from build123d import *

# Parameters (mm, degrees)
SKETCH_2_R      = 1.5
EXTRUDE_1_DEPTH = 1.5
SKETCH_3_R      = 17.5
EXTRUDE_2_DEPTH = 33
SKETCH_4_W      = 21
SKETCH_4_H      = 20
EXTRUDE_3_DEPTH = 15
FILLET_1_R      = 10


with BuildPart() as part:
    # 草图2 → 凸台-拉伸1 (new body)
    with BuildSketch(Plane(origin=(0, 0, 0), x_dir=(1, 0, 0), z_dir=(0, 1, 0))):
        with BuildLine():
            Line((255.573084798, 167.040097328), (242.323084798, 167.040097328))
            Line((242.323084798, 167.040097328), (234.323084798, 159.040097328))
            Line((234.323084798, 159.040097328), (234.323084798, 157.622673023))
            ThreePointArc((234.323084798, 157.622673023), (236.506384931, 155.778710115), (237.323084798, 153.040097328))
            ThreePointArc((237.323084798, 153.040097328), (236.506384931, 150.30148454), (234.323084798, 148.457521633))
            Line((234.323084798, 148.457521633), (234.323084798, 144.040097328))
            Line((234.323084798, 144.040097328), (237.323084798, 144.040097328))
            Line((237.323084798, 144.040097328), (237.323084798, 108.040097328))
            Line((237.323084798, 108.040097328), (234.323084798, 108.040097328))
            Line((234.323084798, 108.040097328), (234.323084798, 104.622673023))
            ThreePointArc((234.323084798, 104.622673023), (236.506384931, 102.778710115), (237.323084798, 100.040097328))
            ThreePointArc((237.323084798, 100.040097328), (236.506384931, 97.30148454), (234.323084798, 95.457521633))
            Line((234.323084798, 95.457521633), (234.323084798, 89.040097328))
            Line((234.323084798, 89.040097328), (254.323084798, 63.040097328))
            Line((254.323084798, 63.040097328), (273.323084798, 63.040097328))
            Line((273.323084798, 63.040097328), (271.323084798, 81.040097328))
            Line((271.323084798, 81.040097328), (291.434195909, 83.040097328))
            Line((291.434195909, 83.040097328), (294.323084798, 57.040097328))
            Line((294.323084798, 57.040097328), (324.323084798, 57.040097328))
            Line((324.323084798, 57.040097328), (327.211973687, 83.040097328))
            Line((327.211973687, 83.040097328), (347.323084798, 81.040097328))
            Line((347.323084798, 81.040097328), (345.323084798, 63.040097328))
            Line((345.323084798, 63.040097328), (364.323084798, 63.040097328))
            Line((364.323084798, 63.040097328), (384.323084798, 89.040097328))
            Line((384.323084798, 89.040097328), (384.323084798, 95.457521633))
            ThreePointArc((384.323084798, 95.457521633), (381.323084798, 100.040097328), (384.323084798, 104.622673023))
            Line((384.323084798, 104.622673023), (384.323084798, 108.040097328))
            Line((384.323084798, 108.040097328), (381.323084798, 108.040097328))
            Line((381.323084798, 108.040097328), (381.323084798, 144.040097328))
            Line((381.323084798, 144.040097328), (384.323084798, 144.040097328))
            Line((384.323084798, 144.040097328), (384.323084798, 148.457521633))
            ThreePointArc((384.323084798, 148.457521633), (381.323084798, 153.040097328), (384.323084798, 157.622673023))
            Line((384.323084798, 157.622673023), (384.323084798, 159.040097328))
            Line((384.323084798, 159.040097328), (376.323084798, 167.040097328))
            Line((376.323084798, 167.040097328), (363.073084798, 167.040097328))
            Line((363.073084798, 167.040097328), (363.073084798, 164.040097328))
            Line((363.073084798, 164.040097328), (327.073084798, 164.040097328))
            Line((327.073084798, 164.040097328), (327.073084798, 167.040097328))
            Line((327.073084798, 167.040097328), (320.573084798, 167.040097328))
            Line((320.573084798, 167.040097328), (320.573084798, 164.040097328))
            Line((320.573084798, 164.040097328), (298.073084798, 164.040097328))
            Line((298.073084798, 164.040097328), (298.073084798, 167.040097328))
            Line((298.073084798, 167.040097328), (291.573084798, 167.040097328))
            Line((291.573084798, 167.040097328), (291.573084798, 164.040097328))
            Line((291.573084798, 164.040097328), (255.573084798, 164.040097328))
            Line((255.573084798, 164.040097328), (255.573084798, 167.040097328))
        make_face()
        with Locations(Location((239.323084798, 105.052003777, 0), (0, 0, 270))):
            Circle(SKETCH_2_R, mode=Mode.SUBTRACT)
        with Locations(Location((379.323084798, 105.052003777, 0), (0, 0, 270))):
            Circle(SKETCH_2_R, mode=Mode.SUBTRACT)
        with Locations(Location((238.323084798, 147.040097328, 0), (0, 0, 270))):
            Circle(SKETCH_2_R, mode=Mode.SUBTRACT)
        with Locations(Location((380.323084798, 147.040097328, 0), (0, 0, 270))):
            Circle(SKETCH_2_R, mode=Mode.SUBTRACT)
    extrude(amount=EXTRUDE_1_DEPTH)

    # 草图3 → 凸台-拉伸2 (add)
    with BuildSketch(Plane(origin=(0, 1.5, 0), x_dir=(1, 0, 0), z_dir=(0, 1, 0))):
        with Locations(Location((275.323084798, 141.040097328, 0), (0, 0, 270))):
            Circle(SKETCH_3_R)
        with Locations(Location((343.323084798, 141.040097328, 0), (0, 0, 270))):
            Circle(SKETCH_3_R)
        with Locations(Location((275.323084798, 105.040097328, 0), (0, 0, 270))):
            Circle(SKETCH_3_R)
        with Locations(Location((343.323084798, 105.040097328, 0), (0, 0, 270))):
            Circle(SKETCH_3_R)
    extrude(amount=EXTRUDE_2_DEPTH)

    # 草图4 → 凸台-拉伸3 (add)
    with BuildSketch(Plane.XZ):
        with Locations((357.823084798, -77.040097328)):
            Rectangle(SKETCH_4_W, SKETCH_4_H)
    extrude(amount=EXTRUDE_3_DEPTH)

    # 圆角1
    # the kernel refuses this fillet: 10 mm, written as the material it takes off along each edge
    with BuildSketch(Plane(origin=(234.323084798, -8.403282896, -159.040097328), x_dir=(0, 0, 1), z_dir=(0, 1, 0))) as fillet_1_piece_1:
        with BuildLine():
            CenterArc((4.694260484, 9.44787514), FILLET_1_R, 225, 25.871759313)
            Line((-2.376807328, 2.376807328), (-2.518228684, 2.235385972))
            Line((-2.518228684, 2.235385972), (-0.141421356, -0.141421356))
            Line((-0.141421356, -0.141421356), (0, -0.2))
            ThreePointArc((0, -0.2), (0.708712153, -0.2), (1.351887581, -0.188957503))
            Line((1.351887581, -0.188957503), (1.417424305, 0))
        make_face()
    extrude(amount=18.306565791, mode=Mode.SUBTRACT)
    with BuildSketch(Plane(origin=(242.323084798, -10.355339059, -167.040097328), x_dir=(-0.7071067811865476, 0, 0.7071067811865476), z_dir=(0, 1, 0)), Plane(origin=(376.323084798, -10.355339059, -167.040097328), x_dir=(-1, 0, 0), z_dir=(0, 1, 0))) as fillet_1_piece_2:
        with BuildLine():
            CenterArc((FILLET_1_R * 0.414213562373, FILLET_1_R), FILLET_1_R, 225, 45)
            Line((-FILLET_1_R * 0.292893218813, FILLET_1_R * 0.292893218813), (-FILLET_1_R * 0.307035354437, FILLET_1_R * 0.27875108319))
            Line((-FILLET_1_R * 0.307035354437, FILLET_1_R * 0.27875108319), (-FILLET_1_R * 0.00828427124746, -FILLET_1_R * 0.02))
            Line((-FILLET_1_R * 0.00828427124746, -FILLET_1_R * 0.02), (FILLET_1_R * 0.414213562373, -FILLET_1_R * 0.02))
            Line((FILLET_1_R * 0.414213562373, -FILLET_1_R * 0.02), (FILLET_1_R * 0.414213562373, 0))
        make_face()
    extrude(amount=22.210678119, mode=Mode.SUBTRACT)
    with BuildSketch(Plane(origin=(384.323084798, -8.403282896, -159.040097328), x_dir=(-0.7071067811865475, 0, -0.7071067811865475), z_dir=(0, 1, 0))) as fillet_1_piece_3:
        with BuildLine():
            CenterArc((3.361313158, 10), FILLET_1_R, 244.128240687, 25.871759313)
            Line((-1.002270338, 1.002270338), (-1.089542008, 0.822315745))
            ThreePointArc((-1.089542008, 0.822315745), (-0.642556525, 0.359713813), (-0.141421356, -0.141421356))
            Line((-0.141421356, -0.141421356), (0, -0.2))
            Line((0, -0.2), (3.361313158, -0.2))
            Line((3.361313158, -0.2), (3.361313158, 0))
        make_face()
    extrude(amount=18.306565791, mode=Mode.SUBTRACT)
    with BuildSketch(Plane(origin=(384.323084798, -8.503048667, -89.040097328), x_dir=(0, 0, -1), z_dir=(0, 1, 0)), Plane(origin=(234.323084798, -8.503048667, -89.040097328), x_dir=(0.6097107608496891, 0, 0.7926239891046025), z_dir=(0, 1, 0))) as fillet_1_piece_4:
        with BuildLine():
            CenterArc((FILLET_1_R * 0.340121946686, FILLET_1_R), FILLET_1_R, 232.431407971, 37.568592029)
            Line((-FILLET_1_R * 0.269588814164, FILLET_1_R * 0.207376010895), (-FILLET_1_R * 0.281783029381, FILLET_1_R * 0.191523531113))
            Line((-FILLET_1_R * 0.281783029381, FILLET_1_R * 0.191523531113), (-FILLET_1_R * 0.00680243893371, -FILLET_1_R * 0.02))
            Line((-FILLET_1_R * 0.00680243893371, -FILLET_1_R * 0.02), (FILLET_1_R * 0.340121946686, -FILLET_1_R * 0.02))
            Line((FILLET_1_R * 0.340121946686, -FILLET_1_R * 0.02), (FILLET_1_R * 0.340121946686, 0))
        make_face()
    extrude(amount=18.506097334, mode=Mode.SUBTRACT)
    with BuildSketch(Plane(origin=(364.323084798, -12.310037436, -63.040097328), x_dir=(0.6097107608496888, 0, -0.792623989104603), z_dir=(0, 1, 0)), Plane(origin=(254.323084798, -12.310037436, -63.040097328), x_dir=(1, 0, 0), z_dir=(0, 1, 0))) as fillet_1_piece_5:
        with BuildLine():
            CenterArc((FILLET_1_R * 0.492401497451, FILLET_1_R), FILLET_1_R, 217.568592029, 52.431407971)
            Line((-FILLET_1_R * 0.300222491654, FILLET_1_R * 0.39028923915), (-FILLET_1_R * 0.316074971436, FILLET_1_R * 0.378095023933))
            Line((-FILLET_1_R * 0.316074971436, FILLET_1_R * 0.378095023933), (-FILLET_1_R * 0.00984802994901, -FILLET_1_R * 0.02))
            Line((-FILLET_1_R * 0.00984802994901, -FILLET_1_R * 0.02), (FILLET_1_R * 0.492401497451, -FILLET_1_R * 0.02))
            Line((FILLET_1_R * 0.492401497451, -FILLET_1_R * 0.02), (FILLET_1_R * 0.492401497451, 0))
        make_face()
    extrude(amount=26.120074873, mode=Mode.SUBTRACT)
    with BuildSketch(Plane(origin=(324.323084798, -22.376069828, -57.040097328), x_dir=(0.1104315260748475, 0, -0.9938837346736189), z_dir=(0, 1, 0)), Plane(origin=(294.323084798, -22.376069828, -57.040097328), x_dir=(1, 0, 0), z_dir=(0, 1, 0))) as fillet_1_piece_6:
        with BuildLine():
            CenterArc((FILLET_1_R * 0.895042793126, FILLET_1_R), FILLET_1_R, 186.340191746, 83.659808254)
            Line((-FILLET_1_R * 0.0988409415472, FILLET_1_R * 0.889568473925), (-FILLET_1_R * 0.118718616241, FILLET_1_R * 0.887359843404))
            Line((-FILLET_1_R * 0.118718616241, FILLET_1_R * 0.887359843404), (-FILLET_1_R * 0.0179008558625, -FILLET_1_R * 0.02))
            Line((-FILLET_1_R * 0.0179008558625, -FILLET_1_R * 0.02), (FILLET_1_R * 0.895042793126, -FILLET_1_R * 0.02))
            Line((FILLET_1_R * 0.895042793126, -FILLET_1_R * 0.02), (FILLET_1_R * 0.895042793126, 0))
        make_face()
    extrude(amount=46.252139656, mode=Mode.SUBTRACT)


solid = part.part
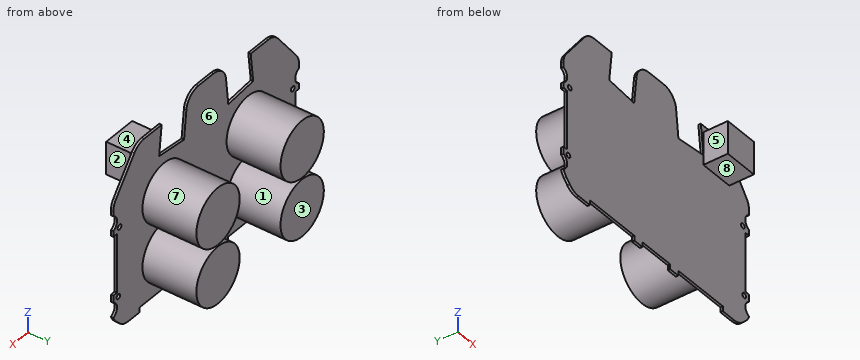
The listing builds one solid part. Answer for the finished solid, in the listing's coordinates (mm). Face numbers are marked on the shaded views. A direction names the side the tool comes from. Coordinates: 2 decimals unless noted, no trailing zeros. Loops run counter-clockwise (first coordinate to the right, second up) from the corner with the lowest first, then second, coordinate; pieces in that order, holes last. Notation, with made-up numbers: (-6.75, -11) -> (14.25, -11) arc R30 ccw to (14.25, 24) -> close; hole circle Ø11 at (50, 30). An arc over 180 degrees is marked (long way). Write item = value, one per line. Start each with the question number.
1) Straight lines are drawn through the part: line 1 (Y direction, x = 262, z = -161.5); line 2 (X direction, y = 2.5, z = -157); line 3 (X direction, y = 5, z = -140). For each, find the intervals that lie inside material, in ascending order. Write a range as from..to.
2) A cutting plane is placed at C-C (y = 8). Give the vertices of the cut face in (x, z), then the cut area to 3 significant figures.
3) A cutting plane is placed at A-A (x = 357.5). Give the vertices of the cut face in (y, z).
4) Given pin 1 Ø0.8 at (x, y) = (235.5, 1) entering from +Z; pin 2 Ø4 at (x, z) = (239.32, -105.05) entering from +Y; pin 3 Ø1.6 at (y, z) = (1, -119) entering from -X, each flat-ended and moving along its own axis, determine where each tip first touches the part or whether it passes through.
5) A cutting plane is placed at D-D (y = -4). Give the vertices of the cut face in (x, z).
6) A tool of negligible diameter and unlimited length cuts with its end or side. For the marked faces 1, 2, 3 and 4, from which of +Z, -Z, +X, -X, +Y, -Y can it reach the whole face along a straight path? Write none if from no direction.
7) A cutting plane is placed at B-B (z = -129). Give the vertices of the cut face in (x, y).
8) The mould has two halves that part along X. Classify the marked faces 5, 6, 7 and 8: released by +X, released by -X, zero draft, split by the parting line, or undercut.
Responses:
q1.line_1 = 0..1.5
q1.line_2 = 268.14..282.5, 336.14..350.5
q1.line_3 = 257.85..292.79, 325.85..360.79
q2.outline = circle Ø35 at (275.32, -141.04); circle Ø35 at (275.32, -105.04); circle Ø35 at (343.32, -141.04); circle Ø35 at (343.32, -105.04)
q2.area = 3,850 mm²
q3.outline = (-15, -87.04) -> (0, -87.04) -> (0, -164.04) -> (1.5, -164.04) -> (1.5, -151.3) -> (34.5, -151.3) -> (34.5, -130.78) -> (1.5, -130.78) -> (1.5, -115.3) -> (34.5, -115.3) -> (34.5, -94.78) -> (1.5, -94.78) -> (1.5, -63.04) -> (0, -63.04) -> (0, -67.04) -> (-15, -67.04) -> close
q4.pin_1 = -87.05
q4.pin_2 = 1.5
q4.pin_3 = 237.32
q5.outline = (347.32, -87.04) -> (368.32, -87.04) -> (368.32, -67.04) -> (347.32, -67.04) -> close
q6.face_1 = +Y
q6.face_2 = +Z, -Z, +X, -Y
q6.face_3 = +Z, -Z, +X, -X, +Y
q6.face_4 = +Z, +X, -X, -Y
q7.outline = (237.32, 0) -> (381.32, 0) -> (381.32, 1.5) -> (356.02, 1.5) -> (356.02, 34.5) -> (330.62, 34.5) -> (330.62, 1.5) -> (288.02, 1.5) -> (288.02, 34.5) -> (262.62, 34.5) -> (262.62, 1.5) -> (237.32, 1.5) -> close
q8.face_5 = released by -X
q8.face_6 = undercut
q8.face_7 = undercut
q8.face_8 = zero draft
